```python
from build123d import *

# Parameters (mm, degrees)
EXTRUDE_THIN1_DEPTH = 190.5
FILLET1_R           = 0.889


with BuildPart() as part:
    # Sketch1 → Extrude-Thin1 (new body)
    with BuildSketch(Plane.XY):
        with BuildLine():
            Line((0, 14.2875), (0, 17.4625))
            Line((0, 17.4625), (-3.175, 17.4625))
            Line((-3.175, 17.4625), (-3.175, 15.08125))
            ThreePointArc((-3.175, 15.08125), (-6.80591832, 15.086090387), (-9.38501075, 12.530337363))
            ThreePointArc((-9.38501075, 12.530337363), (-12.305011444, 8.289373521), (-16.66875, 5.55625))
            Line((-16.66875, 5.55625), (-16.66875, 3.175))
            Line((-16.66875, 3.175), (-19.05, 3.175))
            Line((-19.05, 3.175), (-19.05, 0))
            Line((-19.05, 0), (-15.875, 0))
            Line((-15.875, 0), (-15.875, 0.889))
            Line((-15.875, 0.889), (-18.161, 0.889))
            Line((-18.161, 0.889), (-18.161, 2.286))
            Line((-18.161, 2.286), (-15.77975, 2.286))
            Line((-15.77975, 2.286), (-15.77975, 4.95323652))
            ThreePointArc((-15.77975, 4.95323652), (-11.467396752, 7.865532848), (-8.565790095, 12.185085979))
            ThreePointArc((-8.565790095, 12.185085979), (-5.760091082, 14.478232), (-2.286, 13.448107355))
            Line((-2.286, 13.448107355), (-2.286, 16.5735))
            Line((-2.286, 16.5735), (-0.889, 16.5735))
            Line((-0.889, 16.5735), (-0.889, 14.2875))
            Line((-0.889, 14.2875), (0, 14.2875))
        make_face()
    extrude(amount=-EXTRUDE_THIN1_DEPTH)

    # Fillet1
    fillet1_edges = [part.edges().sort_by_distance(p)[0] for p in [
        (-19.05, 0, -95.25),
        (-19.05, 3.175, -95.25),
        (-16.66875, 5.55625, -95.25),
        (-3.175, 17.4625, -95.25),
        (0, 17.4625, -95.25),
        (-2.286, 13.448107355, -95.25),
        (-15.77975, 2.286, -95.25),
    ]]
    fillet(fillet1_edges, radius=FILLET1_R)


solid = part.part
```
CAD build for the part. Positions are in the model's coordinates, mm. Round coordinates to 2 decimals unless told otherwise and drop trailing zeros. Loops run counter-clockwise (first coordinate to the right, second up) from the corner with the lowest first, then second, coordinate; pieces in that order, holes last. Notation, with made-up numbers: M -4.75,1 L 18.25,1 A12 cw 18.25,16 Z; hole C -1.5,51 d5. An arc over 180 degrees is marked long. Use a Markdown table: item, result. Add a question column.
(1) Drill centre lines: line 1 (Y direction, x = -17.75, z = -134.5) (3 decimals); line 2 (X direction, y = 3.25, z = -108); line 3 (Y direction, x = -2, z = -99). Where is each one in solid material? Low to high.
(2) Flat gauge pins, fed straight in: pin 1 (1.1 mm diameter, centred on x = -17, z = -107.5, fed in from +Y); pin 2 (2.5 mm diameter, centred on y = 15, z = -130, fed in from -X); pin 3 (2 mm diameter, centred on y = 4.5, z = -80, fed in from -X). Where does each tip first touch, or does it go through?
(3) Pull direction X, two halves, no side cores. Call faces 1 (the face through (-11, 9, -190.5)), 2 (the face through (-11.519, 7.814, -93.916)), 3 (the face through (-6.507, 14.247, -93.916)): +X half, -X half, draft (parallel to the pull), parting line (faces both ways), or undercut.
(4) Cut at B-B (x = -6.75). Give the cut face in (y, z).
(5) Cut at C-C (y = 10.5). Give the cut face in (x, z).
Geometry says:
| question | item | result |
|---|---|---|
| 1 | line 1 | y = 0 to 0.889, 2.286 to 3.175 |
| 1 | line 2 | x = -16.67 to -15.78 |
| 1 | line 3 | y = 16.57 to 17.46 |
| 2 | pin 1 | stops at y = 5.54 |
| 2 | pin 2 | stops at x = -8.64 |
| 2 | pin 3 | stops at x = -16.67 |
| 3 | face 1 | draft |
| 3 | face 2 | +X half |
| 3 | face 3 | undercut |
| 4 | outline | M 14.13,-190.5 L 15.11,-190.5 L 15.11,0 L 14.13,0 Z |
| 5 | outline | M -10.47,-190.5 L -9.42,-190.5 L -9.42,0 L -10.47,0 Z |
